from build123d import *

# Parameters (mm, degrees)
SKETCH1_R           = 1.75
SKETCH1_R_2         = 14
BOSS_EXTRUDE1_DEPTH = 7
BOSS_EXTRUDE2_DEPTH = 34
BOSS_EXTRUDE3_DEPTH = 7
CUT_EXTRUDE1_DEPTH  = 41
SKETCH1_2_R         = 14
CUT_EXTRUDE2_DEPTH  = 15


with BuildPart() as part:
    # Sketch1 → Boss-Extrude1 (new body)
    with BuildSketch(Plane(origin=(0, 0, 0), x_dir=(1, 0, 0), z_dir=(0, 1, 0))):
        with BuildLine():
            Line((17.5, -21), (-17.5, -21))
            ThreePointArc((-17.5, -21), (-19.974873734, -19.974873734), (-21, -17.5))
            Line((-21, -17.5), (-21, 17.5))
            ThreePointArc((-21, 17.5), (-19.974873734, 19.974873734), (-17.5, 21))
            Line((-17.5, 21), (17.5, 21))
            ThreePointArc((17.5, 21), (19.974873734, 19.974873734), (21, 17.5))
            Line((21, 17.5), (21, -17.5))
            ThreePointArc((21, -17.5), (19.974873734, -19.974873734), (17.5, -21))
        make_face()
        with Locations((-17.5, -17.5)):
            Circle(SKETCH1_R, mode=Mode.SUBTRACT)
        with Locations((-17.5, 17.5)):
            Circle(SKETCH1_R, mode=Mode.SUBTRACT)
        with Locations((17.5, -17.5)):
            Circle(SKETCH1_R, mode=Mode.SUBTRACT)
        with Locations((17.5, 17.5)):
            Circle(SKETCH1_R, mode=Mode.SUBTRACT)
        Circle(SKETCH1_R_2, mode=Mode.SUBTRACT)
    extrude(amount=BOSS_EXTRUDE1_DEPTH)

    # Sketch2 → Boss-Extrude2 (add)
    with BuildSketch(Plane(origin=(0, 7, 0), x_dir=(1, 0, 0), z_dir=(0, 1, 0))):
        with BuildLine():
            Line((21, -17.5), (21, 17.5))
            ThreePointArc((21, 17.5), (19.974873734, 19.974873734), (17.5, 21))
            Line((17.5, 21), (-17.5, 21))
            ThreePointArc((-17.5, 21), (-19.974873734, 19.974873734), (-21, 17.5))
            Line((-21, 17.5), (-21, -17.5))
            ThreePointArc((-21, -17.5), (-19.974873734, -19.974873734), (-17.5, -21))
            Line((-17.5, -21), (17.5, -21))
            ThreePointArc((17.5, -21), (19.974873734, -19.974873734), (21, -17.5))
        make_face()
    extrude(amount=BOSS_EXTRUDE2_DEPTH)

    # Sketch3 → Boss-Extrude3 (add)
    with BuildSketch(Plane(origin=(0, 41, 0), x_dir=(1, 0, 0), z_dir=(0, 1, 0))):
        with BuildLine():
            Line((17.5, 21), (-17.5, 21))
            ThreePointArc((-17.5, 21), (-19.974873734, 19.974873734), (-21, 17.5))
            Line((-21, 17.5), (-21, -17.5))
            ThreePointArc((-21, -17.5), (-19.974873734, -19.974873734), (-17.5, -21))
            Line((-17.5, -21), (17.5, -21))
            ThreePointArc((17.5, -21), (19.974873734, -19.974873734), (21, -17.5))
            Line((21, -17.5), (21, 17.5))
            ThreePointArc((21, 17.5), (19.974873734, 19.974873734), (17.5, 21))
        make_face()
    extrude(amount=BOSS_EXTRUDE3_DEPTH)

    # Sketch4 → Cut-Extrude1 (cut)
    with BuildSketch(Plane(origin=(0, 48, 0), x_dir=(1, 0, 0), z_dir=(0, 1, 0))):
        with BuildLine():
            Line((-13.8, 13.8), (-18, 13.8))
            Line((-18, 13.8), (-21, 10.8))
            Line((-21, 10.8), (-21, 17.5))
            ThreePointArc((-21, 17.5), (-19.974873734, 19.974873734), (-17.5, 21))
            Line((-17.5, 21), (-10.45, 21))
            Line((-10.45, 21), (-13.8, 17.65))
            Line((-13.8, 17.65), (-13.8, 13.8))
        make_face()
        with BuildLine():
            Line((17.5, 21), (10.45, 21))
            Line((10.45, 21), (13.8, 17.65))
            Line((13.8, 17.65), (13.8, 13.8))
            Line((13.8, 13.8), (18, 13.8))
            Line((18, 13.8), (21, 10.8))
            Line((21, 10.8), (21, 17.5))
            ThreePointArc((21, 17.5), (19.974873734, 19.974873734), (17.5, 21))
        make_face()
        with BuildLine():
            Line((-17.5, -21), (-10.45, -21))
            Line((-10.45, -21), (-13.8, -17.65))
            Line((-13.8, -17.65), (-13.8, -13.8))
            Line((-13.8, -13.8), (-18, -13.8))
            Line((-18, -13.8), (-21, -10.8))
            Line((-21, -10.8), (-21, -17.5))
            ThreePointArc((-21, -17.5), (-19.974873734, -19.974873734), (-17.5, -21))
        make_face()
        with BuildLine():
            Line((21, -17.5), (21, -10.8))
            Line((21, -10.8), (18, -13.8))
            Line((18, -13.8), (13.8, -13.8))
            Line((13.8, -13.8), (13.8, -17.65))
            Line((13.8, -17.65), (10.45, -21))
            Line((10.45, -21), (17.5, -21))
            ThreePointArc((17.5, -21), (19.974873734, -19.974873734), (21, -17.5))
        make_face()
    extrude(amount=-CUT_EXTRUDE1_DEPTH, mode=Mode.SUBTRACT)

    # Sketch1_2 → Cut-Extrude2 (cut)
    with BuildSketch(Plane(origin=(0, 0, 0), x_dir=(1, 0, 0), z_dir=(0, 1, 0))):
        Circle(SKETCH1_2_R)
    extrude(amount=CUT_EXTRUDE2_DEPTH, mode=Mode.SUBTRACT)


solid = part.part
Geometry: final body of the model. Coordinates: model frame, mm. A direction names the side the tool comes from. Coordinates: 2 decimals unless noted, no trailing zeros. Loops run counter-clockwise (first coordinate to the right, second up) from the corner with the lowest first, then second, coordinate; pieces in that order, holes last. Notation, with made-up numbers: M 58.25,80.5 L 94.25,80.5 A10 cw 94.25,95.5 Z; hole C 7,12 d7. An arc over 180 degrees is marked long. One line per item, written item: value. Start each with the question number.
1) Draft query along Z for faces 6 (the cylindrical face through (17.272, 3.451, 15.765)), 7 (the flat face through (15.7, 7, -18.2)), 8 (the flat face through (19.5, 27.8, -12.3)), 9 (the flat face through (0, 24, 21)). Return one class per face: released by +Z, released by -Z, zero draft, split by the parting line, or undercut.
2) Reachability of faces 1 (the flat face through (0, 15, 0)), 2 (the flat face through (-13.8, 28, -16)), 3 (the flat face through (12.15, 27.79, 19.3)), 4 (the flat face through (-19.5, 27.8, 12.3)), 5 (the flat face through (13.8, 28, -16)) from +Z, -Z, +X, -X, +Y, -Y: full face, straight path, thin tool, end or side. Return the list, or none.
3) Cut plane A-A (y = 5). Return loops of the section in (x, z).
4) Cut plane B-B (z = 15). Return loops of the section in (x, y).
5) Cut plane D-D (y = 41). Return loops of the section in (x, z).
6) Material intervals for L1, parallel to Z at x = 17.5, y = 2.75; L2, parallel to Z at x = 0, y = 8.75, sorted ascending. Write a range as from..to.
7) Cut plane C-C (x = -1.5). Return loops of the section in (y, z).
8) Pin query (flat end, axial travel): P1, Ø4, axis at x = -17.5, z = 17.5, coming from the +Y side; P2, Ø4, axis at y = 29.5, z = -15, coming from the -X side; P3, Ø3.5, axis at x = -15.5, y = 25.5, coming from the +Z side. Return the tip coordinate at first contact, or that it passes through.
Evaluation:
1. face 6: undercut
1. face 7: zero draft
1. face 8: released by -Z
1. face 9: released by +Z
2. face 1: -Y
2. face 2: -Z, -X, +Y
2. face 3: +Z, +X, +Y
2. face 4: +Z, -X, +Y
2. face 5: -Z, +X, +Y
3. outline: M -21,-17.5 A3.5 ccw -17.5,-21 L 17.5,-21 A3.5 ccw 21,-17.5 L 21,17.5 A3.5 ccw 17.5,21 L -17.5,21 A3.5 ccw -21,17.5 Z; hole C -17.5,-17.5 d3.5; hole C -17.5,17.5 d3.5; hole C 0,0 d28; hole C 17.5,-17.5 d3.5; hole C 17.5,17.5 d3.5
4. outline: M -21,0 L 21,0 L 21,7 L 13.8,7 L 13.8,48 L -13.8,48 L -13.8,7 L -21,7 Z
5. outline: M -21,-10.8 L -18,-13.8 L -13.8,-13.8 L -13.8,-17.65 L -10.45,-21 L 10.45,-21 L 13.8,-17.65 L 13.8,-13.8 L 18,-13.8 L 21,-10.8 L 21,10.8 L 18,13.8 L 13.8,13.8 L 13.8,17.65 L 10.45,21 L -10.45,21 L -13.8,17.65 L -13.8,13.8 L -18,13.8 L -21,10.8 Z
6. L1: -21..-19.25, -15.75..15.75, 19.25..21
6. L2: -21..-14, 14..21
7. outline: M 0,-21 L 48,-21 L 48,21 L 0,21 L 0,13.92 L 15,13.92 L 15,-13.92 L 0,-13.92 Z
8. P1: y = 7
8. P2: x = -18.8
8. P3: z = 17.7
